Here's how the part is built. I have some questions about the finished solid (model axes, mm). A direction names the side the tool comes from. Round coordinates to 2 decimals unless told otherwise and drop trailing zeros. Loops run counter-clockwise (first coordinate to the right, second up) from the corner with the lowest first, then second, coordinate; pieces in that order, holes last. Notation, with made-up numbers: M 38.5,-28.75 L 53.5,-28.75 A24 ccw 53.5,-2.75 Z; hole C 44,24 d4. An arc over 180 degrees is marked long. Use a Markdown table: item, result.
```python
from build123d import *

# Parameters (mm, degrees)
SALIENTE_EXTRUIR1_DEPTH = 8.5
REDONDEO1_R             = 2
CORTAR_EXTRUIR1_START   = -10
CORTAR_EXTRUIR1_DEPTH   = 10
CROQUIS3_W              = 2
CROQUIS3_H              = 37.641018094
CORTAR_EXTRUIR2_DEPTH   = 10
CROQUIS4_W              = 20.360825868
CROQUIS4_H              = 3.8
CORTAR_EXTRUIR3_DEPTH   = 10
REDONDEO2_R             = 1
REDONDEO3_R             = 2
CORTAR_EXTRUIR4_DEPTH   = 10
CORTAR_EXTRUIR5_DEPTH   = 10
REDONDEO4_R             = 2
CROQUIS9_W              = 0.360825868
CROQUIS9_H              = 41.677341087
CORTAR_EXTRUIR6_DEPTH   = 10
CROQUIS10_W             = 14.5
CROQUIS10_H             = 0.285488866
SALIENTE_EXTRUIR2_DEPTH = 8.5


with BuildPart() as part:
    # Croquis1 → Saliente-Extruir1 (new body)
    with BuildSketch(Plane(origin=(0, 0, 0), x_dir=(1, 0, 0), z_dir=(0, 1, 0))):
        with BuildLine():
            Line((13.270197773, -14.714511134), (13.270197773, -24.714511134))
            Line((13.270197773, -24.714511134), (28.270197773, -24.714511134))
            Line((28.270197773, -24.714511134), (28.270197773, 24.714511134))
            Line((28.270197773, 24.714511134), (13.270197773, 24.714511134))
            Line((13.270197773, 24.714511134), (13.270197773, 14.714511134))
            Line((13.270197773, 14.714511134), (-6.590628095, 14.714511134))
            ThreePointArc((-6.590628095, 14.714511134), (-6.944181486, 14.860957744), (-7.090628095, 15.214511134))
            Line((-7.090628095, 15.214511134), (-7.090628095, 18.995462915))
            ThreePointArc((-7.090628095, 18.995462915), (-7.383521314, 19.702569696), (-8.090628095, 19.995462915))
            ThreePointArc((-8.090628095, 19.995462915), (-12.706365951, 18.287755027), (-16.090628095, 14.714511134))
            Line((-16.090628095, 14.714511134), (-16.090628095, 10.714511134))
            Line((-16.090628095, 10.714511134), (13.270197773, 10.714511134))
            Line((13.270197773, 10.714511134), (13.270197773, 8.214511134))
            Line((13.270197773, 8.214511134), (13.270197773, 5.212235466))
            Line((13.270197773, 5.212235466), (13.270197773, 5.012235466))
            Line((13.270197773, 5.012235466), (13.270197773, 3.012235466))
            Line((13.270197773, 3.012235466), (-16.090628095, 3.012235466))
            Line((-16.090628095, 3.012235466), (-16.090628095, -3.012235466))
            Line((-16.090628095, -3.012235466), (13.270197773, -3.012235466))
            Line((13.270197773, -3.012235466), (13.270197773, -5.012235466))
            Line((13.270197773, -5.012235466), (13.270197773, -5.212235466))
            Line((13.270197773, -5.212235466), (13.270197773, -8.214511134))
            Line((13.270197773, -8.214511134), (13.270197773, -10.714511134))
            Line((13.270197773, -10.714511134), (-16.090628095, -10.714511134))
            Line((-16.090628095, -10.714511134), (-16.090628095, -14.714511134))
            ThreePointArc((-16.090628095, -14.714511134), (-12.706365951, -18.287755027), (-8.090628095, -19.995462915))
            ThreePointArc((-8.090628095, -19.995462915), (-7.383521314, -19.702569696), (-7.090628095, -18.995462915))
            Line((-7.090628095, -18.995462915), (-7.090628095, -14.714511134))
            Line((-7.090628095, -14.714511134), (13.270197773, -14.714511134))
        make_face()
    extrude(amount=SALIENTE_EXTRUIR1_DEPTH)

    # Redondeo1
    redondeo1_edges = [part.edges().sort_by_distance(p)[0] for p in [
        (13.270197773, 4.25, -14.714511134),
        (13.270197773, 4.25, 14.714511134),
    ]]
    fillet(redondeo1_edges, radius=REDONDEO1_R)

    # Croquis2 → Cortar-Extruir1 (cut)
    with BuildSketch(Plane(origin=(0, 8.5, 0), x_dir=(1, 0, 0), z_dir=(0, 1, 0)).offset(CORTAR_EXTRUIR1_START)):
        with BuildLine():
            Line((-7.090628095, 18.995462915), (-7.090628095, 17.354987025))
            ThreePointArc((-7.090628095, 17.354987025), (-11.747603416, 16.569795769), (-16.090628095, 14.714511134))
            ThreePointArc((-16.090628095, 14.714511134), (-12.706365951, 18.287755027), (-8.090628095, 19.995462915))
            ThreePointArc((-8.090628095, 19.995462915), (-7.383521314, 19.702569696), (-7.090628095, 18.995462915))
        make_face()
        with BuildLine():
            Line((-7.090628095, -18.995462915), (-7.090628095, -17.354987025))
            ThreePointArc((-7.090628095, -17.354987025), (-11.747603416, -16.569795769), (-16.090628095, -14.714511134))
            ThreePointArc((-16.090628095, -14.714511134), (-12.706365951, -18.287755027), (-8.090628095, -19.995462915))
            ThreePointArc((-8.090628095, -19.995462915), (-7.383521314, -19.702569696), (-7.090628095, -18.995462915))
        make_face()
    extrude(amount=CORTAR_EXTRUIR1_DEPTH, mode=Mode.SUBTRACT)

    # Croquis3 → Cortar-Extruir2 (cut)
    with BuildSketch(Plane(origin=(0, 8.5, 0), x_dir=(1, 0, 0), z_dir=(0, 1, 0))):
        with Locations((-15.090628095, -0.838537532)):
            Rectangle(CROQUIS3_W, CROQUIS3_H)
    extrude(amount=-CORTAR_EXTRUIR2_DEPTH, mode=Mode.SUBTRACT)

    # Croquis4 → Cortar-Extruir3 (cut)
    with BuildSketch(Plane(origin=(0, 8.5, 0), x_dir=(1, 0, 0), z_dir=(0, 1, 0))):
        with Locations((3.089784839, 15.454987025)):
            Rectangle(CROQUIS4_W, CROQUIS4_H)
        with Locations((3.089784839, -15.454987025)):
            Rectangle(CROQUIS4_W, CROQUIS4_H)
    extrude(amount=-CORTAR_EXTRUIR3_DEPTH, mode=Mode.SUBTRACT)

    # Redondeo2
    redondeo2_edges = [part.edges().sort_by_distance(p)[0] for p in [
        (-7.090628095, 4.25, -13.554987025),
        (-7.090628095, 4.25, 13.554987025),
    ]]
    fillet(redondeo2_edges, radius=REDONDEO2_R)

    # Redondeo3
    redondeo3_edges = [part.edges().sort_by_distance(p)[0] for p in [
        (13.270197773, 4.25, -13.554987025),
        (13.270197773, 4.25, 13.554987025),
    ]]
    fillet(redondeo3_edges, radius=REDONDEO3_R)

    # Croquis6 → Cortar-Extruir4 (cut)
    with BuildSketch(Plane(origin=(0, 8.5, 0), x_dir=(1, 0, 0), z_dir=(0, 1, 0))):
        Polygon((-14.090628095, -3.012235466), (13.270197773, -3.012235466), (13.270197773, -2.512235466), (-13.590628095, -2.512235466), (-13.590628095, 2.512235466), (13.270197773, 2.512235466), (13.270197773, 3.012235466), (-14.090628095, 3.012235466), align=None)
    extrude(amount=-CORTAR_EXTRUIR4_DEPTH, mode=Mode.SUBTRACT)

    # Croquis7 → Cortar-Extruir5 (cut)
    with BuildSketch(Plane(origin=(0, 8.5, 0), x_dir=(1, 0, 0), z_dir=(0, 1, 0))):
        Polygon((13.270197773, 24.714511134), (13.770197773, 24.714511134), (13.770197773, 13.554987025), (13.270197773, 13.554987025), (10.850472816, 13.554987025), (10.850472816, 24.714511134), align=None)
        Polygon((13.270197773, -24.714511134), (10.850472816, -24.714511134), (10.850472816, -13.554987025), (13.270197773, -13.554987025), (13.770197773, -13.554987025), (13.770197773, -24.714511134), align=None)
    extrude(amount=-CORTAR_EXTRUIR5_DEPTH, mode=Mode.SUBTRACT)

    # Redondeo4
    redondeo4_edges = [part.edges().sort_by_distance(p)[0] for p in [
        (13.770197773, 4.25, -13.554987025),
        (13.770197773, 4.25, 13.554987025),
    ]]
    fillet(redondeo4_edges, radius=REDONDEO4_R)

    # Croquis9 → Cortar-Extruir6 (cut)
    with BuildSketch(Plane(origin=(0, 8.5, 0), x_dir=(1, 0, 0), z_dir=(0, 1, 0))):
        with Locations((-13.910215161, 4.161329456)):
            Rectangle(CROQUIS9_W, CROQUIS9_H)
    extrude(amount=-CORTAR_EXTRUIR6_DEPTH, mode=Mode.SUBTRACT)

    # Croquis10 → Saliente-Extruir2 (add)
    with BuildSketch(Plane(origin=(0, 8.5, 0), x_dir=(1, 0, 0), z_dir=(0, 1, 0))):
        with Locations((21.020197773, 24.857255567)):
            Rectangle(CROQUIS10_W, CROQUIS10_H)
        with Locations((21.020197773, -24.857255567)):
            Rectangle(CROQUIS10_W, CROQUIS10_H)
    extrude(amount=-SALIENTE_EXTRUIR2_DEPTH)


solid = part.part
```
Q1. Will these pins go through, and if not, where does the flat tip stop? P1, Ø2.5, axis at x = -4, y = 3, coming from the -Z side (3 decimals); P2, Ø4, axis at y = 2.5, z = 5.5, coming from the -X side; P3, Ø1, axis at x = 9, z = 8.5, coming from the -Y side; P4, Ø4, axis at x = 2.5, y = 5, coming from the +Z side (3 decimals).
Return value:
| item | result |
|---|---|
| P1 | stops at z = -13.555 |
| P2 | stops at x = 13.27 |
| P3 | passes through |
| P4 | stops at z = 13.555 |
Q2. Imagine slicing it at C-C, the plane x = -11. Please give me the cut outline in (y, z), then the cut area to 3 significant figures.
Return value:
| item | result |
|---|---|
| outline | M 0,-16.77 L 8.5,-16.77 L 8.5,-10.71 L 0,-10.71 Z; M 0,-2.51 L 8.5,-2.51 L 8.5,2.51 L 0,2.51 Z; M 0,10.71 L 8.5,10.71 L 8.5,16.77 L 0,16.77 Z |
| area | 146 mm^2 |
Q3. I need wall thicknesses on line 1 (Z direction, x = 0, y = 5.5); line 2 (Z direction, x = -8.5, y = 7.5); line 3 (X direction, y = 8, z = 0.5). Which ranges of each line are inside material? Lowest first, please. Write a range as from..to.
Return value:
| item | result |
|---|---|
| line 1 | z = -13.55..-10.71, -2.51..2.51, 10.71..13.55 |
| line 2 | z = -17.24..-10.71, -2.51..2.51, 10.71..17.24 |
| line 3 | x = -13.59..28.27 |
Q4. We'd pull the mould along X, two halves only. Please class faces 5 (the flat face through (-13.73, 4, -13)), 6 (the flat face through (0, 4, 2.512)), 7 (the cylindrical face through (-6.79, 4.19, 13.84)): pulls with the +X half, pulls with the -X half, needs draft (parallel to the pull), parting line crosses it, or undercut.
Return value:
| item | result |
|---|---|
| face 5 | pulls with the -X half |
| face 6 | needs draft |
| face 7 | undercut |
Q5. For faces 1 (the flat face through (13.27, 4, -7)), 2 (the flat face through (13.77, 4, 20)), 3 (the cylindrical face through (-10, 4, 17)), 4 (the cylindrical face through (-6.81, 4.19, -13.86)), which set-ups out of +Z, -Z, +X, -X, +Y, -Y let a thin tool reach every point of the face, with its end or its side?
Return value:
| item | result |
|---|---|
| face 1 | -X, +Y, -Y |
| face 2 | +Z, +Y, -Y |
| face 3 | +Z, -X, +Y, -Y |
| face 4 | -Z, +Y, -Y |
Q6. Imagine slicing it at A-A, the plane x = -3. Please give me the cut outline in (y, z).
Return value:
| item | result |
|---|---|
| outline | M 0,-13.55 L 8.5,-13.55 L 8.5,-10.71 L 0,-10.71 Z; M 0,-2.51 L 8.5,-2.51 L 8.5,2.51 L 0,2.51 Z; M 0,10.71 L 8.5,10.71 L 8.5,13.55 L 0,13.55 Z |
Q7. Imagine slicing it at B-B, the plane y = 6.5. Please give me the cut outline in (x, z), then the cut area to 3 significant figures.
Return value:
| item | result |
|---|---|
| outline | M -13.73,-15.87 A20 ccw -7.09,-17.35 L -7.09,-14.55 A1 cw -6.09,-13.55 L 11.77,-13.55 A2 cw 13.77,-15.55 L 13.77,-25 L 28.27,-25 L 28.27,25 L 13.77,25 L 13.77,15.55 A2 cw 11.77,13.55 L -6.09,13.55 A1 cw -7.09,14.55 L -7.09,17.35 A20 ccw -13.73,15.87 L -13.73,10.71 L 13.27,10.71 L 13.27,2.51 L -13.59,2.51 L -13.59,-2.51 L 13.27,-2.51 L 13.27,-10.71 L -13.73,-10.71 Z |
| area | 1,070 mm^2 |
Q8. Imagine slicing it at D-D, the plane z = -18. Please give me the cut outline in (x, y).
Return value:
| item | result |
|---|---|
| outline | M 13.77,0 L 28.27,0 L 28.27,8.5 L 13.77,8.5 Z |
